Autodesk Inventor part; units mm, degrees
ref_plane "YZ Plane" through (0, 0, 0) normal (1, 0, 0) x (0, 1, 0)
ref_plane "XZ Plane" through (0, 0, 0) normal (0, 1, 0) x (-1, 0, 0)
ref_plane "XY Plane" through (0, 0, 0) normal (0, 0, 1) x (1, 0, 0)
sketch "Sketch1" plane through (0, 0, 0) normal (0, 0, 1) x (1, 0, 0)
  line L0 (0, 0) -> (300, 0)
  line L1 (300, 0) -> (300, 300)
  line L2 (300, 300) -> (0, 300)
  line L3 (0, 300) -> (0, 0)
  dimension "d0" = 300
  dimension "d1" = 300
extrude "Extrusion1" add sketch "Sketch1" along normal blind 3.175
sketch "Sketch2" plane through (0, 0, 3.175) normal (0, 0, 1) x (1, 0, 0)
  line L0 (0, 300) -> (0, 0)
  line L1 (300, 300) -> (0, 300)
  line L2 (300, 0) -> (300, 300)
  line L3 (0, 0) -> (300, 0)
  point P0 (7, 293)
  point P1 (293, 293)
  point P2 (293, 7)
  point P3 (7, 7)
  dimension "d4" = 7
  dimension "d5" = 7
  dimension "d6" = 7
  dimension "d7" = 7
  dimension "d8" = 7
  dimension "d9" = 7
  dimension "d10" = 7
  dimension "d11" = 7
hole "Hole1" at (7, 293, 3.175) at (293, 293, 3.175) at (293, 7, 3.175) at (7, 7, 3.175) direction (0, 0, -1) diameter 8 depth 25.4 tip angle 118
sketch "Sketch3" plane through (0, 0, 3.175) normal (0, 0, 1) x (1, 0, 0)
  line L0 (0, 300) -> (0, 0)
  line L1 (0, 0) -> (300, 0)
  line L2 (300, 0) -> (300, 300)
  point P0 (46, 254)
  point P1 (254, 254)
  point P2 (254, 46)
  point P3 (46, 46)
  dimension "d19" = 208
  dimension "d20" = 208
  dimension "d21" = 208
  dimension "d22" = 46
  dimension "d23" = 46
  dimension "d24" = 46
  dimension "d25" = 208
  dimension "d26" = 46
hole "Hole2" at (46, 254, 3.175) at (254, 254, 3.175) at (254, 46, 3.175) at (46, 46, 3.175) direction (0, 0, -1) diameter 3 depth 25.4 tip angle 118
sketch "Sketch4" plane through (0, 0, 3.175) normal (0, 0, 1) x (1, 0, 0)
  line L0 (0, 0) -> (300, 0)
  line L1 (0, 300) -> (0, 0)
  line L2 (300, 0) -> (300, 300)
  line L3 (300, 300) -> (0, 300)
  point P0 (150, 7)
  point P1 (293, 150)
  point P2 (150, 293)
  point P3 (7, 150)
  dimension "d34" = 150
  dimension "d35" = 7
  dimension "d36" = 7
  dimension "d37" = 150
  dimension "d38" = 7
  dimension "d39" = 7
  dimension "d40" = 150
  dimension "d41" = 150
hole "Hole3" at (150, 7, 3.175) at (293, 150, 3.175) at (150, 293, 3.175) at (7, 150, 3.175) direction (0, 0, -1) diameter 8 depth 25.4 tip angle 118
properties part number "bed plate square"
Read the model definition and answer for the solid it produces. Units are mm, in the model's axes. Give positions to 0.01 mm unless a question says otherwise; leave off trailing zeros. Write each loop counter-clockwise with the first axis right and the second up, starting at its lowest first coordinate (ties: lowest second). Pieces come first, ordered by that corner, then holes. Notation, with made-up numbers: (20, 30) - (72, 30) arc R16 cw to (72, 58) - close; hole circle Ø10 at (65.25, 82.25). An arc over 180 degrees is marked (long way). Write item = value, one per line. Start each with the question number.
Item 1: Find section B-B (y = 150). Give the vertices of the cut face in (x, z) (3 decimals).
Item 2: The mould has two halves that part along Y. Classify faces 1 (the cylindrical face through (146.034, 7.521, 1.565)), 2 (the flat face through (148, 152, 3.175)), 3 (the cylindrical face through (7, 297, 2)): +Y half, -Y half, draft (parallel to the pull), parting line (faces both ways), or undercut.
Item 3: Find the intervals of material crossed by probe 1 along Y at (x, z) = (150, 2.2); probe 2 along Y at (x, z) = (46, 2.2); probe 3 along Y at (x, z) = (293, 1.05), in increasing order. Write a range as [from, to].
Item 4: Each of these flat-tipped pins is pushed along its axis until it touches: P1, Ø9, axis at x = 7, y = 293, coming from the -Z side; P2, Ø6.5, axis at x = 293, y = 150, coming from the +Z side. Where does it stop, or does it pass through?
Item 5: Find section A-A (x = 293). Give the vertices of the cut face in (y, z) (3 decimals), then the cut area to 3 significant figures.
Response:
q1.outline = (0, 0) - (3, 0) - (3, 3.175) - (0, 3.175) - close; (11, 0) - (289, 0) - (289, 3.175) - (11, 3.175) - close; (297, 0) - (300, 0) - (300, 3.175) - (297, 3.175) - close
q2.face_1 = undercut
q2.face_2 = draft
q2.face_3 = undercut
q3.probe_1 = [0, 3], [11, 289], [297, 300]
q3.probe_2 = [0, 44.5], [47.5, 252.5], [255.5, 300]
q3.probe_3 = [0, 3], [11, 146], [154, 289], [297, 300]
q4.P1 = 0
q4.P2 = through
q5.outline = (0, 0) - (3, 0) - (3, 3.175) - (0, 3.175) - close; (11, 0) - (146, 0) - (146, 3.175) - (11, 3.175) - close; (154, 0) - (289, 0) - (289, 3.175) - (154, 3.175) - close; (297, 0) - (300, 0) - (300, 3.175) - (297, 3.175) - close
q5.area = 876 mm²
